from build123d import *

# Parameters (mm, degrees)
SKIZZE1_W                        = 35
SKIZZE1_H                        = 75
AUFSATZ_LINEAR_AUSTRAGEN1_DEPTH  = 1.5
SKIZZE3_W                        = 15.25
SKIZZE3_H                        = 5
SKIZZE3_W_2                      = 4.875
SCHNITT_LINEAR_AUSTRAGEN12_DEPTH = 20
SCHNITT_LINEAR_AUSTRAGEN15_DEPTH = 1.5
SKIZZE9_W                        = 1
SKIZZE9_H                        = 5.796251951
AUFSATZ_LINEAR_AUSTRAGEN6_DEPTH  = 1.5


with BuildPart() as part:
    # Skizze1 → Aufsatz-Linear austragen1 (new body)
    with BuildSketch(Plane.XY):
        with Locations((17.5, 37.5)):
            Rectangle(SKIZZE1_W, SKIZZE1_H)
    extrude(amount=AUFSATZ_LINEAR_AUSTRAGEN1_DEPTH)

    # Skizze3 → Schnitt-Linear austragen12 (cut)
    with BuildSketch(Plane.XY.offset(1.5)):
        with Locations((17.5, 2.5)):
            Rectangle(SKIZZE3_W, SKIZZE3_H)
        with Locations((32.5625, 2.5)):
            Rectangle(SKIZZE3_W_2, SKIZZE3_H)
        with Locations((2.4375, 2.5)):
            Rectangle(SKIZZE3_W_2, SKIZZE3_H)
    extrude(amount=-SCHNITT_LINEAR_AUSTRAGEN12_DEPTH, mode=Mode.SUBTRACT)

    # Skizze8 → Schnitt-Linear austragen15 (cut)
    with BuildSketch(Plane.XY.offset(1.5)):
        Polygon((5.5, 32.342192337), (24.167481122, 64.5), (25.167481122, 64.5), (25.167481122, 32.342192337), (29.5, 32.342192337), (29.5, 31.342192337), (25.167481122, 31.342192337), (25.167481122, 17), (24.167481122, 17), (24.167481122, 31.342192337), (5.5, 31.342192337), align=None)
        Polygon((6.5, 32.342192337), (24.167481122, 32.342192337), (24.167481122, 62.777335466), align=None, mode=Mode.SUBTRACT)
    extrude(amount=-SCHNITT_LINEAR_AUSTRAGEN15_DEPTH, mode=Mode.SUBTRACT)


with BuildPart() as schnitt_linear_austragen15_piece_1:
    # of the separate pieces the step leaves, piece 1, a body of its own (schnitt_linear_austragen15_pieces)
    add(part.part.solids().sort_by_distance((4.875, 0, 0))[0])



with BuildPart() as schnitt_linear_austragen15_piece_2:
    # of the separate pieces the step leaves, piece 2, a body of its own (schnitt_linear_austragen15_pieces)
    add(part.part.solids().sort_by_distance((24.167481122, 62.777335466, 0))[0])


with BuildPart() as schnitt_linear_austragen15_piece_1_1:
    add(schnitt_linear_austragen15_piece_1.part)

    add(schnitt_linear_austragen15_piece_2.part)  # Aufsatz-Linear austragen6 merges Schnitt-Linear austragen15 piece 2
    # Skizze9 → Aufsatz-Linear austragen6 (add)
    with BuildSketch(Plane.XY.offset(1.5)):
        with Locations((15.327481122, 31.334841656)):
            Rectangle(SKIZZE9_W, SKIZZE9_H)
    extrude(amount=-AUFSATZ_LINEAR_AUSTRAGEN6_DEPTH)


solid = schnitt_linear_austragen15_piece_1_1.part
The model under review builds one solid part; all positions refer to its coordinate system, in mm. A direction names the side the tool comes from. Round coordinates to 2 decimals unless told otherwise and drop trailing zeros. Order: outer loops, then holes, each group sorted by start corner. A loop starts at its lowest first (then second) coordinate and runs counter-clockwise, first axis right, second up. Notation, with made-up numbers: (74.25, -5.75) -> (131.25, -5.75) arc R27 ccw to (131.25, 12.25) -> close; hole circle Ø11 at (58, -3). An arc over 180 degrees is marked (long way). Write item = value, one per line. Start each with the question number.
Item 1: For line 1 along Y through (x, z) = (27.5, 0.6); line 2 along Y through (x, z) = (11, 0.9); line 3 along X through (y, z) = (57, 0.35), list the stretches that pass through material, from the lowest coordinate up.
Item 2: For faces 1 (the face through (35, 40, 1)), 2 (the face through (27, 32.342, 1)), 3 (the face through (4.875, 2, 1)), 4 (the face through (17, 5, 1)), 5 (the face through (30.125, 2, 1)), list the 3-axis set-ups (+Z, -Z, +X, -X, +Y, -Y) from which the entire face can be reached by the end or side of a thin tool; tool diameter is ignored.
Item 3: Mouldability with a two-part tool opening along Y and no side actions: class faces 6 (the face through (9.875, 2, 1)), 7 (the face through (7, 0, 1)), 8 (the face through (20, 31.342, 1)) as released by +Y, released by -Y, zero draft, split by the parting line, or undercut.
Item 4: Consider section B-B on x = 23. Write out the cut boundary in (y, z), plus the area to 3 significant figures.
Item 5: Consider section A-A on y = 29.5. Write out the cut boundary in (x, z), plus the area to 3 significant figures.
Item 6: Consider section D-D on y = 57. Write out the cut boundary in (x, z), plus the area to 3 significant figures.
Item 7: Clearance check with a flat-ended pin moving along its axis: pin 1 Ø0.8 at (x, z) = (18.5, 1) entering from -Y. State where the tip first meets the part, or that it passes through.
Conclusion:
q1.line_1 = 0 to 31.34, 32.34 to 75
q1.line_2 = 5 to 31.34, 32.34 to 40.09, 41.82 to 75
q1.line_3 = 0 to 19.81, 20.81 to 24.17, 25.17 to 35
q2.face_1 = +Z, -Z, +X, +Y, -Y
q2.face_2 = +Z, -Z
q2.face_3 = +Z, -Z, -X, -Y
q2.face_4 = +Z, -Z, -Y
q2.face_5 = +Z, -Z, +X, -Y
q3.face_6 = zero draft
q3.face_7 = released by -Y
q3.face_8 = undercut
q4.outline = (5, 0) -> (31.34, 0) -> (31.34, 1.5) -> (5, 1.5) -> close; (32.34, 0) -> (60.77, 0) -> (60.77, 1.5) -> (32.34, 1.5) -> close; (62.49, 0) -> (75, 0) -> (75, 1.5) -> (62.49, 1.5) -> close
q4.area = 101 mm2
q5.outline = (0, 0) -> (24.17, 0) -> (24.17, 1.5) -> (0, 1.5) -> close; (25.17, 0) -> (35, 0) -> (35, 1.5) -> (25.17, 1.5) -> close
q5.area = 51.0 mm2
q6.outline = (0, 0) -> (19.81, 0) -> (19.81, 1.5) -> (0, 1.5) -> close; (20.81, 0) -> (24.17, 0) -> (24.17, 1.5) -> (20.81, 1.5) -> close; (25.17, 0) -> (35, 0) -> (35, 1.5) -> (25.17, 1.5) -> close
q6.area = 49.5 mm2
q7.pin_1 = 5
